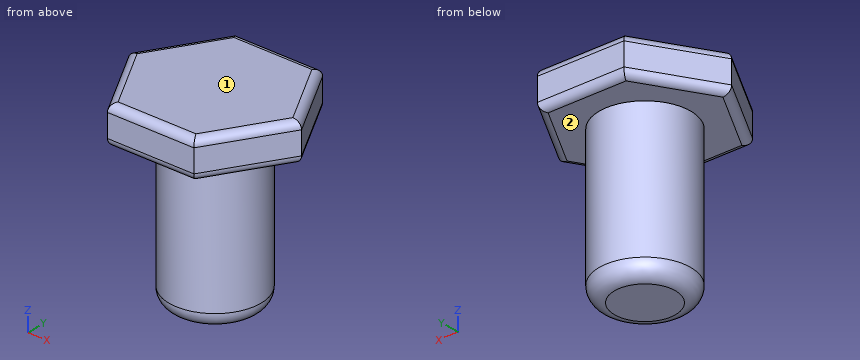
```python
from build123d import *

# Parameters (mm, degrees)
SKETCH_1_R      = 6
EXTRUDE_1_DEPTH = 20
EXTRUDE_2_DEPTH = 5
FILLET_1_R      = 2
FILLET_2_R      = 1


with BuildPart() as part:
    # 草图1 → 凸台-拉伸1 (new body)
    with BuildSketch(Plane.XY):
        Circle(SKETCH_1_R)
    extrude(amount=EXTRUDE_1_DEPTH)

    # 草图2 → 凸台-拉伸2 (add)
    with BuildSketch(Plane.XY.offset(20)):
        Polygon((5.773502692, -10), (11.547005384, 0), (5.773502692, 10), (-5.773502692, 10), (-11.547005384, 0), (-5.773502692, -10), align=None)
    extrude(amount=EXTRUDE_2_DEPTH)

    # 圆角1
    fillet_1_edges = [part.edges().sort_by_distance(p)[0] for p in [
        (-6, 0, 0),
    ]]
    fillet(fillet_1_edges, radius=FILLET_1_R)

    # 圆角2
    fillet_2_edges = [part.edges().sort_by_distance(p)[0] for p in [
        (0, -10, 20),
        (8.660254038, -5, 20),
        (8.660254038, 5, 20),
        (0, 10, 20),
        (-8.660254038, 5, 20),
        (-8.660254038, -5, 20),
        (0, -10, 25),
        (8.660254038, -5, 25),
        (8.660254038, 5, 25),
        (0, 10, 25),
        (-8.660254038, 5, 25),
        (-8.660254038, -5, 25),
    ]]
    fillet(fillet_2_edges, radius=FILLET_2_R)


solid = part.part
```
The model under review builds one solid part; all positions refer to its coordinate system, in mm. Face numbers are marked on the shaded views. A direction names the side the tool comes from. Round coordinates to 2 decimals unless told otherwise and drop trailing zeros. Order: outer loops, then holes, each group sorted by start corner. A loop starts at its lowest first (then second) coordinate and runs counter-clockwise, first axis right, second up.
Item 1: For pin 1 (8 mm diameter, centred on x = -3, z = 15.5, fed in from +Y); pin 2 (2 mm diameter, centred on y = 5, z = 3.5, fed in from -X); pin 3 (4 mm diameter, centred on y = -5.5, z = 22.5, fed in from +X); pin 4 (9 mm diameter, centred on x = -4.5, y = 3.5, fed in from -Z), all flat-tipped, find the tip position at first contact; note any pin that passes through.
Working result:
pin 1: stops at y = 6
pin 2: stops at x = -4.47
pin 3: stops at x = 9.53
pin 4: stops at z = 0
Item 2: Add section A-A, the plane z = 23. State the section outline as (x, y) points, and give its area (3 significant figures).
Working result:
outline: (-11.55, 0) - (-5.77, -10) - (5.77, -10) - (11.55, 0) - (5.77, 10) - (-5.77, 10) - close
area: 346 mm2
Item 3: Machinability: for the marked faces 1 and 2, which of the approach directions +Z, -Z, +X, -X, +Y, -Y give a long, thin tool a straight path to every point of the face, cutting with its end or side? Answer none if there is none.
Working result:
face 1: +Z, +X, -X, +Y, -Y
face 2: -Z
Item 4: Add section C-C, the plane z = 13. State the section outline as (x, y) points.
Working result:
outline: circle Ø12 at (0, 0)
Item 5: Add section B-B, the plane x = 0. State the section outline as (y, z) points.
Working result:
outline: (-10, 21) arc R1 ccw to (-9, 20) - (-6, 20) - (-6, 2) arc R2 ccw to (-4, 0) - (4, 0) arc R2 ccw to (6, 2) - (6, 20) - (9, 20) arc R1 ccw to (10, 21) - (10, 24) arc R1 ccw to (9, 25) - (-9, 25) arc R1 ccw to (-10, 24) - close
Item 6: To check wall thickness, follow probe 1 along Z at (x, y) = (-3.5, -5); probe 2 along X at (y, z) = (-3, 12); probe 3 along Y at (x, z) = (0.25, 11). State the ranges of each line that lie inside material, in increasing order.
Working result:
probe 1: z = 20 to 25
probe 2: x = -5.2 to 5.2
probe 3: y = -5.99 to 5.99
